from build123d import *

# Parameters (mm, degrees)
SKETCH_1_R      = 1.75
SKETCH_1_R_2    = 5
EXTRUDE_1_DEPTH = 2
FILLET_1_R      = 3
EXTRUDE_START   = -2
SKETCH_2_R      = 5
SKETCH_2_R_2    = 2.7
EXTRUDE_2_DEPTH = 2
EXTRUDE_3_DEPTH = 2


with BuildPart() as part:
    # 草图1 → 凸台-拉伸1 (new body)
    with BuildSketch(Plane(origin=(0, 0, 0), x_dir=(1, 0, 0), z_dir=(0, 1, 0))):
        with BuildLine():
            Line((0, 27), (0, 0))
            Line((0, 0), (42, 0))
            ThreePointArc((42, 0), (43.414213562, 0.585786438), (44, 2))
            Line((44, 2), (44, 13))
            ThreePointArc((44, 13), (43.414213562, 14.414213562), (42, 15))
            Line((42, 15), (29.5, 15))
            Line((29.5, 15), (29.5, 21))
            ThreePointArc((29.5, 21), (27.01040764, 27.01040764), (21, 29.5))
            Line((21, 29.5), (0, 27))
        make_face()
        with Locations(Location((22, 7.5, 0), (0, 0, 270))):
            Circle(SKETCH_1_R, mode=Mode.SUBTRACT)
        with Locations(Location((37, 7.5, 0), (0, 0, 270))):
            Circle(SKETCH_1_R, mode=Mode.SUBTRACT)
        with Locations(Location((7.5, 22, 0), (0, 0, 270))):
            Circle(SKETCH_1_R, mode=Mode.SUBTRACT)
        with Locations(Location((21, 21, 0), (0, 0, 270))):
            Circle(SKETCH_1_R_2, mode=Mode.SUBTRACT)
    extrude(amount=EXTRUDE_1_DEPTH)

    # 圆角1
    fillet_1_edges = [part.edges().sort_by_distance(p)[0] for p in [
        (29.5, 1, -15),
    ]]
    fillet(fillet_1_edges, radius=FILLET_1_R)

    # 草图2 → 凸台-拉伸2 (add)
    with BuildSketch(Plane(origin=(0, 2, 0), x_dir=(1, 0, 0), z_dir=(0, 1, 0)).offset(EXTRUDE_START)):
        with Locations((21, 21)):
            Circle(SKETCH_2_R)
        with Locations(Location((21, 21, 0), (0, 0, 270))):
            Circle(SKETCH_2_R_2, mode=Mode.SUBTRACT)
    extrude(amount=EXTRUDE_2_DEPTH)

    # 草图3 → 凸台-拉伸3 (add)
    with BuildSketch(Plane(origin=(0, 2, 0), x_dir=(1, 0, 0), z_dir=(0, 1, 0))):
        Polygon((21, 29.5), (0, 29.5), (0, 27), align=None)
    extrude(amount=-EXTRUDE_3_DEPTH)


solid = part.part
Check sheet for the modelled part. Datum: model origin and axes. Units: mm. A direction names the side the tool comes from. Give positions to 0.01 mm unless a question says otherwise; leave off trailing zeros. Loops run counter-clockwise (first coordinate to the right, second up) from the corner with the lowest first, then second, coordinate; pieces in that order, holes last. Notation, with made-up numbers: M -4,32.5 L 48,32.5 A16 ccw 48,41.5 Z; hole C -5.5,59 d8. An arc over 180 degrees is marked long. Use a Markdown table: item, result. Add a question column.
Q1. Tool access check on faces 1 (the flat face through (37, 1, -15)), 2 (the flat face through (11, 1, -29.5)). Record the directions out of +Z, -Z, +X, -X, +Y, -Y that give a thin tool (end or side, any length) a straight path to the whole face; none if there is none.
Q2. Go/stop test with flat-tipped pins: pin 1 (3 mm diameter, centred on x = 39, z = -17, fed in from +Y); pin 2 (1 mm diameter, centred on y = 1, z = -19.5, fed in from +X). Record where each tip stops, or that it passes through.
Q3. Sectioned sample at B-B, the plane x = 37. Record the cut outline in (y, z).
Q4. Sectioned sample at D-D, the plane x = 22. Record the cut outline in (y, z).
Q5. Sectioned sample at C-C, the plane y = 1.5. Record the cut outline in (x, z).
Q6. Mould release check, pull along X, two halves, no side actions. Record for faces 3 (the cylindrical face through (23.677, 0.986, -21.351)), 4 (the flat face through (17, 2, -12)), 5 (the flat face through (0, 1, -15)): pulls with the +X half, pulls with the -X half, needs draft (parallel to the pull), parting line crosses it, or undercut.
Q7. Sectioned sample at A-A, the plane z = -7.5. Record the cut outline in (x, y), then the cut area to 3 significant figures.
Q8. Scan lines: line 1 along X through (y, z) = (0.8, -7.5); line 2 along X through (y, z) = (1, -21); line 3 along X through (y, z) = (0.4, -17.75). Record each from-to range of solid material in increasing order. Write a range as [from, to].
Verdict:
| question | item | result |
|---|---|---|
| 1 | face 1 | -Z, +X, +Y, -Y |
| 1 | face 2 | -Z, +X, -X, +Y, -Y |
| 2 | pin 1 | through |
| 2 | pin 2 | x = 29.5 |
| 3 | outline | M 0,-15 L 2,-15 L 2,-9.25 L 0,-9.25 Z; M 0,-5.75 L 2,-5.75 L 2,0 L 0,0 Z |
| 4 | outline | M 0,-29.44 L 2,-29.44 L 2,-23.51 L 0,-23.51 Z; M 0,-18.49 L 2,-18.49 L 2,-9.25 L 0,-9.25 Z; M 0,-5.75 L 2,-5.75 L 2,0 L 0,0 Z |
| 5 | outline | M 0,-29.5 L 21,-29.5 A8.5 ccw 29.5,-21 L 29.5,-18 A3 cw 32.5,-15 L 42,-15 A2 ccw 44,-13 L 44,-2 A2 ccw 42,0 L 0,0 Z; hole C 7.5,-22 d3.5; hole C 21,-21 d5.4; hole C 22,-7.5 d3.5; hole C 37,-7.5 d3.5 |
| 6 | face 3 | undercut |
| 6 | face 4 | needs draft |
| 6 | face 5 | pulls with the -X half |
| 7 | outline | M 0,0 L 20.25,0 L 20.25,2 L 0,2 Z; M 23.75,0 L 35.25,0 L 35.25,2 L 23.75,2 Z; M 38.75,0 L 44,0 L 44,2 L 38.75,2 Z |
| 7 | area | 74.0 mm^2 |
| 8 | line 1 | [0, 20.25], [23.75, 35.25], [38.75, 44] |
| 8 | line 2 | [0, 6.06], [8.94, 18.3], [23.7, 29.5] |
| 8 | line 3 | [0, 29.51] |
